Design review of the part built by this model. Coordinates are the model's own, in mm. A direction names the side the tool comes from. Coordinates: 2 decimals unless noted, no trailing zeros. Write each loop counter-clockwise with the first axis right and the second up, starting at its lowest first coordinate (ties: lowest second). Pieces come first, ordered by that corner, then holes.
Q1. For probe 1 along X at (y, z) = (4.6, 23.5); probe 2 along X at (y, z) = (5, 24); probe 3 along Y at (x, z) = (7.25, 24.5), list the stretches that pass through material, from the lowest coordinate up.
Q2. Take a section at B-B (y = 9). Give the boundary of the cut face in (x, z).
Q3. Machinability: for faces 4 (the flat face through (12.5, 3.539, 4.9)), 5 (the flat face through (2.6, 3.505, 6.8)), 6 (the cylindrical face through (0.285, 3.33, 33.699)), 7 (the flat face through (7, 3, 34)), which of the approach directions +Z, -Z, +X, -X, +Y, -Y give a long, thin tool a straight path to every point of the face, cutting with its end or side? Answer none if there is none.
Q4. Take a section at A-A (x = 11.1). Give the boundary of the cut face in (y, z).
Q5. Mouldability with a two-part tool opening along X and no side actions: class faces 1 (the flat face through (7, 9, 43)), 2 (the flat face through (12.5, 3.539, 24.9)), 3 (the cylindrical face through (0.301, 3.315, 0.285)) as pulls with the +X half, pulls with the -X half, needs draft (parallel to the pull), parting line crosses it, or undercut.
Q6. Insertion check: pin 1 (1.5 mm diameter, centred on x = 11, z = 20, fed in from +Y); pin 2 (4 mm diameter, centred on x = 8.5, y = 8.5, fed in from -Z); pin 3 (3 mm diameter, centred on x = 12.5, z = 23.5, fed in from +Y); pin 4 (2 mm diameter, centred on x = 6, y = 3.5, fed in from +Z). Each pin has a flat end and moves straight along its axis. Give the tip position at first contact, or say it passes through.
Q7. Take a section at D-D (x = 4.5). Give the boundary of the cut face in (y, z).
Q8. Take a section at C-C (z = 23.5). Give the boundary of the cut face in (x, y), and give its area (3 significant figures).
```python
from build123d import *

# Parameters (mm, degrees)
SKETCH1_W                                      = 15
SKETCH1_H                                      = 6.539
BOSS_EXTRUDE1_DEPTH                            = 30
CBORE_FOR_M3_SHCS1_D                           = 3.6
CBORE_FOR_M3_SHCS1_CBORE_D                     = 6.5
CBORE_FOR_M3_SHCS1_CBORE_DEPTH                 = 3
CBORE_FOR_6_SOCKET_HEAD_CAP_SCREW1_D           = 3.997300108
CBORE_FOR_6_SOCKET_HEAD_CAP_SCREW1_CBORE_D     = 7.14502
CBORE_FOR_6_SOCKET_HEAD_CAP_SCREW1_CBORE_DEPTH = 3.5052
BOSS_EXTRUDE2_DEPTH                            = 15
FILLET1_R                                      = 1


with BuildPart() as part:
    # Sketch1 → Boss-Extrude1 (new body)
    with BuildSketch(Plane.XY):
        with Locations((7.5, 3.2695)):
            Rectangle(SKETCH1_W, SKETCH1_H)
    extrude(amount=BOSS_EXTRUDE1_DEPTH)

    # CBORE for M3 SHCS1 (through all)
    with Locations(Plane(origin=(0, 6.539, 0), x_dir=(1, 0, 0), z_dir=(0, 1, 0))):
        with Locations((11.1, -3.5), (11.1, -23.5)):
            CounterBoreHole(CBORE_FOR_M3_SHCS1_D / 2, CBORE_FOR_M3_SHCS1_CBORE_D / 2, CBORE_FOR_M3_SHCS1_CBORE_DEPTH)

    # CBORE for #6 Socket Head Cap Screw1 (through all)
    with Locations(Plane(origin=(0, 0, 0), x_dir=(-1, 0, 0), z_dir=(0, -1, 0))):
        with Locations((-4.175, -24.779), (-4.175, -5.221)):
            CounterBoreHole(CBORE_FOR_6_SOCKET_HEAD_CAP_SCREW1_D / 2, CBORE_FOR_6_SOCKET_HEAD_CAP_SCREW1_CBORE_D / 2, CBORE_FOR_6_SOCKET_HEAD_CAP_SCREW1_CBORE_DEPTH)

    # Sketch6 → Boss-Extrude2 (add)
    with BuildSketch(Plane.ZY):
        Polygon((30, 0), (34, 0), (34, 6.569), (43, 6.569), (43, 11.569), (30, 11.569), align=None)
    extrude(amount=-BOSS_EXTRUDE2_DEPTH)

    # Fillet1
    fillet1_edges = [part.edges().sort_by_distance(p)[0] for p in [
        (0, 9.054, 30),
        (0, 3.2845, 34),
        (0, 9.069, 43),
        (15, 9.054, 30),
        (15, 9.069, 43),
        (15, 3.2845, 34),
        (15, 3.2695, 0),
        (0, 3.2695, 0),
    ]]
    fillet(fillet1_edges, radius=FILLET1_R)


solid = part.part
```
Response:
1. probe 1: x = 0 to 2.64, 5.71 to 7.85, 14.35 to 15
1. probe 2: x = 0 to 2.33, 6.02 to 7.89, 14.31 to 15
1. probe 3: y = 3.51 to 6.54
2. outline: (0, 31) arc R1 ccw to (1, 30) - (14, 30) arc R1 ccw to (15, 31) - (15, 42) arc R1 ccw to (14, 43) - (1, 43) arc R1 ccw to (0, 42) - close
3. face 4: +Y
3. face 5: -Y
3. face 6: +Z, -X, -Y
3. face 7: +Z, +X, -X, -Y
4. outline: (0, 0) - (6.54, 0) - (6.54, 0.25) - (3.54, 0.25) - (3.54, 1.7) - (0, 1.7) - close; (0, 5.3) - (3.54, 5.3) - (3.54, 6.75) - (6.54, 6.75) - (6.54, 20.25) - (3.54, 20.25) - (3.54, 21.7) - (0, 21.7) - close; (0, 25.3) - (3.54, 25.3) - (3.54, 26.75) - (6.54, 26.75) - (6.54, 30) - (11.57, 30) - (11.57, 43) - (6.57, 43) - (6.57, 34) - (0, 34) - close
5. face 1: needs draft
5. face 2: undercut
5. face 3: pulls with the -X half
6. pin 1: stops at y = 6.54
6. pin 2: stops at z = 0
6. pin 3: stops at y = 3.54
6. pin 4: stops at z = 34
7. outline: (0, 0) - (6.54, 0) - (6.54, 3.25) - (3.51, 3.25) - (3.51, 1.66) - (0, 1.66) - close; (0, 8.78) - (3.51, 8.78) - (3.51, 7.19) - (6.54, 7.19) - (6.54, 22.81) - (3.51, 22.81) - (3.51, 21.22) - (0, 21.22) - close; (0, 28.34) - (3.51, 28.34) - (3.51, 26.75) - (6.54, 26.75) - (6.54, 30) - (11.57, 30) - (11.57, 43) - (6.57, 43) - (6.57, 34) - (0, 34) - close
8. outline: (0, 0) - (0.84, 0) - (0.84, 3.51) - (2.64, 3.51) - (2.64, 6.54) - (0, 6.54) - close; (5.71, 3.51) - (7.51, 3.51) - (7.51, 0) - (9.3, 0) - (9.3, 3.54) - (7.85, 3.54) - (7.85, 6.54) - (5.71, 6.54) - close; (12.9, 0) - (15, 0) - (15, 6.54) - (14.35, 6.54) - (14.35, 3.54) - (12.9, 3.54) - close
8. area: 33.1 mm2
